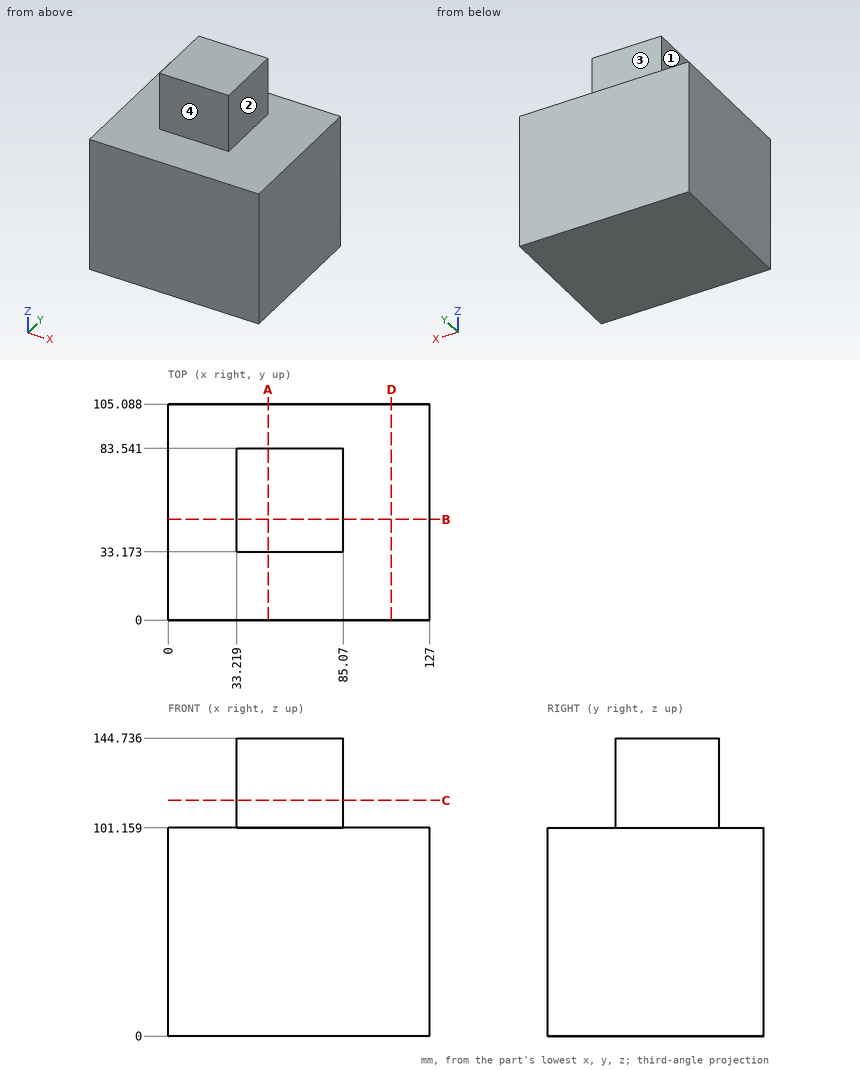
Geometry: see drawing. Coordinates: mm, zero at the bounding-box minimum. A direction names the side the tool comes from. Round coordinates to 2 decimals unless told otherwise and drop trailing zeros. Loops run counter-clockwise (first coordinate to the right, second up) from the corner with the lowest first, then second, coordinate; pieces in that order, holes last. Notation, with made-up numbers: (39, 51.5) -> (55, 51.5) arc R25 cw to (55, 80.5) -> close; hole circle Ø10 at (-2, -36). An arc over 180 degrees is marked (long way). One line per question, with ' | ' between items. Start each with the question number.
1. Line query: line 1 along Z through (x, y) = (79.5, 92.5); line 2 along X through (y, z) = (54, 117); line 3 along Y through (x, z) = (34, 124). Output: solid intervals per line, ascending. Write a range as [from, to].
2. Section B-B on y = 49. Output: boundary loops of the cut face in (x, z) (1 decimal), and give its area (3 significant figures).
3. Section D-D on x = 108.5. Output: boundary loops of the cut face in (y, z).
4. Contact query for flat-ended pins moving along their axis: pin 1 (5 mm diameter, centred on y = 46.5, z = 123.5, fed in from +X); pin 2 (10 mm diameter, centred on x = 104, y = 35, fed in from +Z). Output: stop coordinate, or through.
5. Section C-C on z = 114.5. Output: boundary loops of the cut face in (x, y), and give its area (3 significant figures).
6. Section A-A on x = 48.5. Output: boundary loops of the cut face in (y, z) (1 decimal), and give its area (3 significant figures).
7. Set-up query: the marked faces 1, 2, 3 and 4. Return all of +Z, -Z, +X, -X, +Y, -Y with unobstructed straight access to the full face (end or side cutting, diameter ignored); none if empty.
Returned:
1) line 1: z = [0, 101.16] | line 2: x = [33.22, 85.07] | line 3: y = [33.17, 83.54]
2) outline: (0, 0) -> (127, 0) -> (127, 101.2) -> (85.1, 101.2) -> (85.1, 144.7) -> (33.2, 144.7) -> (33.2, 101.2) -> (0, 101.2) -> close | area: 15,100 mm2
3) outline: (0, 0) -> (105.09, 0) -> (105.09, 101.16) -> (0, 101.16) -> close
4) pin 1: stops at x = 85.07 | pin 2: stops at z = 101.16
5) outline: (33.22, 33.17) -> (85.07, 33.17) -> (85.07, 83.54) -> (33.22, 83.54) -> close | area: 2,610 mm2
6) outline: (0, 0) -> (105.1, 0) -> (105.1, 101.2) -> (83.5, 101.2) -> (83.5, 144.7) -> (33.2, 144.7) -> (33.2, 101.2) -> (0, 101.2) -> close | area: 12,800 mm2
7) face 1: +Z, -X, +Y, -Y | face 2: +Z, +X, +Y, -Y | face 3: +Z, +X, -X, +Y | face 4: +Z, +X, -X, -Y
